Part model, mm, in its own coordinate system. A direction names the side the tool comes from. Coordinates: 2 decimals unless noted, no trailing zeros. Loops run counter-clockwise (first coordinate to the right, second up) from the corner with the lowest first, then second, coordinate; pieces in that order, holes last. Notation, with made-up numbers: (17, 51.25) -> (29, 51.25) arc R25 ccw to (29, 73.25) -> close; hole circle Ø1 at (53.25, 12.5). An arc over 180 degrees is marked (long way). Use one line per item in the form item = value. Start each with the question number.
(1) Pin check, flat tips, straight feed: P1, Ø1.5, axis at y = -4, z = 2.5, coming from the -X side; P2, Ø1.1, axis at y = -6.5, z = 2, coming from the -X side; P3, Ø6, axis at x = 0.5, y = -0.5, coming from the -Z side; P4, Ø0.9, axis at x = 5.5, z = 1.5, coming from the -Y side. Stop position of each tip, or through.
(2) Drill centre lines: L1, parallel to X at y = -6.75, z = 2.8; L2, parallel to X at y = -1.25, z = 1.95; L3, parallel to X at y = -2.25, z = 1.8. Where is each one in solid material? Low to high. Write a range as [from, to].
(3) Mould opens along Y. For faces 1 (the flat face through (35.617, -8, 1)), 2 (the flat face through (-36, -2, 1)), 3 (the flat face through (33, 1, 1)) say: +Y half, -Y half, draft (parallel to the pull), parting line (faces both ways), or undercut.
(4) 3-axis set-ups, long thin cutter, end or side, ignore diameter. For faces 4 (the flat face through (-32, -8, 1)), 5 (the flat face through (20, -2, 1)), 6 (the flat face through (-31.383, -3, 1)): which of +Z, -Z, +X, -X, +Y, -Y reach the whole face in a straight line?
(5) Band-saw the part on C-C on x = -3.5. Give the cut face in (y, z), then the cut area to 3 significant figures.
(6) Band-saw the part on B-B on y = -10.5. Give the cut face in (x, z), then the cut area to 3 significant figures.
```python
from build123d import *

# Parameters (mm, degrees)
BOSS_EXTRUDE1_DEPTH = 3


with BuildPart() as part:
    # Sketch3 → Boss-Extrude1 (new body)
    with BuildSketch(Plane.XY):
        with BuildLine():
            Line((29.616597331, 4), (-41.383402669, 4))
            Line((-41.383402669, 4), (-41.383402669, 1))
            Line((-41.383402669, 1), (-41.383402669, -2))
            Line((-41.383402669, -2), (-31.383402669, -2))
            Line((-31.383402669, -2), (-31.383402669, -5))
            Line((-31.383402669, -5), (-35.383402669, -5))
            ThreePointArc((-35.383402669, -5), (-36.09050945, -5.292893219), (-36.383402669, -6))
            Line((-36.383402669, -6), (-36.383402669, -7))
            ThreePointArc((-36.383402669, -7), (-36.09050945, -7.707106781), (-35.383402669, -8))
            Line((-35.383402669, -8), (-29.383402669, -8))
            ThreePointArc((-29.383402669, -8), (-28.676295888, -7.707106781), (-28.383402669, -7))
            Line((-28.383402669, -7), (-28.383402669, -3))
            ThreePointArc((-28.383402669, -3), (-28.09050945, -2.292893219), (-27.383402669, -2))
            Line((-27.383402669, -2), (6.616597331, -2))
            Line((6.616597331, -2), (6.616597331, -5))
            Line((6.616597331, -5), (2.616597331, -5))
            ThreePointArc((2.616597331, -5), (1.90949055, -5.292893219), (1.616597331, -6))
            Line((1.616597331, -6), (1.616597331, -7))
            ThreePointArc((1.616597331, -7), (1.90949055, -7.707106781), (2.616597331, -8))
            Line((2.616597331, -8), (8.616597331, -8))
            ThreePointArc((8.616597331, -8), (9.323704112, -7.707106781), (9.616597331, -7))
            Line((9.616597331, -7), (9.616597331, -3))
            ThreePointArc((9.616597331, -3), (9.90949055, -2.292893219), (10.616597331, -2))
            Line((10.616597331, -2), (30.616597331, -2))
            Line((30.616597331, -2), (30.616597331, 0))
            ThreePointArc((30.616597331, 0), (30.90949055, 0.707106781), (31.616597331, 1))
            Line((31.616597331, 1), (34.616597331, 1))
            ThreePointArc((34.616597331, 1), (35.323704112, 0.707106781), (35.616597331, 0))
            Line((35.616597331, 0), (35.616597331, -16))
            Line((35.616597331, -16), (40.616597331, -16))
            Line((40.616597331, -16), (40.616597331, 4))
            Line((40.616597331, 4), (35.616597331, 4))
            Line((35.616597331, 4), (29.616597331, 4))
        make_face()
    extrude(amount=BOSS_EXTRUDE1_DEPTH)


solid = part.part
```
A:
q1.P1 = -31.38
q1.P2 = -36.38
q1.P3 = 0
q1.P4 = -8
q2.L1 = [-36.38, -28.38], [1.62, 9.62], [35.62, 40.62]
q2.L2 = [-41.38, 30.62], [35.62, 40.62]
q2.L3 = [-31.38, -28.04], [6.62, 9.96], [35.62, 40.62]
q3.face_1 = draft
q3.face_2 = undercut
q3.face_3 = -Y half
q4.face_4 = +Z, -Z, -X, -Y
q4.face_5 = +Z, -Z, -Y
q4.face_6 = +Z, -Z, -X
q5.outline = (-2, 0) -> (4, 0) -> (4, 3) -> (-2, 3) -> close
q5.area = 18.0 mm²
q6.outline = (35.62, 0) -> (40.62, 0) -> (40.62, 3) -> (35.62, 3) -> close
q6.area = 15.0 mm²
